Work out the finished part from the listing and answer in its coordinate system (mm). Face numbers are marked on the shaded views. A direction names the side the tool comes from. Round coordinates to 2 decimals unless told otherwise and drop trailing zeros. Order: outer loops, then holes, each group sorted by start corner. A loop starts at its lowest first (then second) coordinate and runs counter-clockwise, first axis right, second up. Notation, with made-up numbers: M 61.5,28.5 L 97.5,28.5 A22 ccw 97.5,58.5 Z; hole C 46,11 d11. An arc over 180 degrees is marked long. Return JSON: item names as keys, results as strings.
from build123d import *

# Parameters (mm, degrees)
SKETCH_1_R               = 14.75
EXTRUDE_1_DEPTH          = 20
SKETCH_2_R               = 14
EXTRUDE_2_DEPTH          = 5
SKETCH_3_R               = 14.75
EXTRUDE_3_DEPTH          = 5
SKETCH_4_R               = 14.25
SKETCH_4_R_2             = 13.5
EXTRUDE_4_DEPTH          = 6.7
SKETCH_5_R               = 13.5
EXTRUDE_5_DEPTH          = 6
SKETCH_6_W               = 1
SKETCH_6_H               = 10.048644724
CUT_EXTRUDE_1_DEPTH      = 15
PATTERN_CIRCULAR_1_COUNT = 24
SKETCH_7_R               = 1.5
EXTRUDE_6_DEPTH          = 17.7
SKETCH_8_R               = 10
EXTRUDE_7_DEPTH          = 1
SKETCH_9_R               = 13
EXTRUDE_8_DEPTH          = 3
SKETCH_10_R              = 8.9
EXTRUDE_9_DEPTH          = 3.3


with BuildPart() as part:
    # 草图1 → 凸台-拉伸1 (new body)
    with BuildSketch(Plane(origin=(0, 0, 0), x_dir=(0, 0, -1), z_dir=(1, 0, 0))):
        Circle(SKETCH_1_R)
    extrude(amount=EXTRUDE_1_DEPTH)

    # 草图2 → 凸台-拉伸2 (add)
    with BuildSketch(Plane(origin=(20, 0, 0), x_dir=(0, 0, -1), z_dir=(1, 0, 0))):
        Circle(SKETCH_2_R)
    extrude(amount=EXTRUDE_2_DEPTH)

    # 草图3 → 凸台-拉伸3 (add)
    with BuildSketch(Plane(origin=(25, 0, 0), x_dir=(0, 0, -1), z_dir=(1, 0, 0))):
        Circle(SKETCH_3_R)
    extrude(amount=EXTRUDE_3_DEPTH)

    # 草图4 → 凸台-拉伸4 (add)
    with BuildSketch(Plane(origin=(30, 0, 0), x_dir=(0, 0, -1), z_dir=(1, 0, 0))):
        Circle(SKETCH_4_R)
        Circle(SKETCH_4_R_2, mode=Mode.SUBTRACT)
    extrude(amount=EXTRUDE_4_DEPTH)

    # 草图5 → 凸台-拉伸5 (add)
    with BuildSketch(Plane(origin=(30, 0, 0), x_dir=(0, 0, -1), z_dir=(1, 0, 0))):
        Circle(SKETCH_5_R)
    extrude(amount=EXTRUDE_5_DEPTH)

    # 草图6 → 切除-拉伸1 (cut)
    with BuildSketch(Plane(origin=(36, 0, 0), x_dir=(0, 0, -1), z_dir=(1, 0, 0))):
        with Locations((0, 19.524322362)):
            Rectangle(SKETCH_6_W, SKETCH_6_H)
    cut_extrude_1 = extrude(amount=-CUT_EXTRUDE_1_DEPTH, mode=Mode.SUBTRACT)

    # 阵列(圆周)1: 切除-拉伸1 ×24 about axis
    pattern_circular_1_axis = Axis((0, 0, 0), (1, 0, 0))
    for i in range(1, PATTERN_CIRCULAR_1_COUNT):
        add(cut_extrude_1.rotate(pattern_circular_1_axis, i * 360 / PATTERN_CIRCULAR_1_COUNT), mode=Mode.SUBTRACT)

    # 草图7 → 凸台-拉伸6 (add)
    with BuildSketch(Plane(origin=(0, 0, 0), x_dir=(1, 0, 0), z_dir=(0, 1, 0))):
        with Locations(Location((3.8, 0, 0), (0, 0, 90))):
            Circle(SKETCH_7_R)
        with Locations(Location((16, 0, 0), (0, 0, 90))):
            Circle(SKETCH_7_R)
    extrude(amount=EXTRUDE_6_DEPTH)

    # 草图8 → 凸台-拉伸7 (add)
    with BuildSketch(Plane.ZY):
        Circle(SKETCH_8_R)
    extrude(amount=EXTRUDE_7_DEPTH)

    # 草图9 → 凸台-拉伸8 (add)
    with BuildSketch(Plane.ZY.offset(1)):
        Circle(SKETCH_9_R)
    extrude(amount=EXTRUDE_8_DEPTH)

    # 草图10 → 凸台-拉伸9 (add)
    with BuildSketch(Plane.ZY.offset(4)):
        Circle(SKETCH_10_R)
    extrude(amount=EXTRUDE_9_DEPTH)


solid = part.part
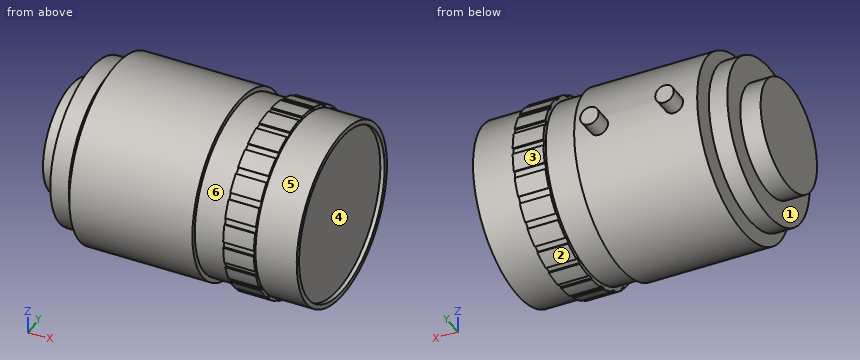
Item 1: Consider line 1 along Y through (x, z) = (36.35, 0); line 2 along X through (y, z) = (-10.5, 3.75); line 3 along X through (y, z) = (3, 6). Determine where each line is inside the solid, lowest interval first. Write a range as [from, to].
Output:
{"line 1": "y = [-14.25, -13.5], [13.5, 14.25]", "line 2": "x = [-4, -1], [0, 36]", "line 3": "x = [-7.3, 36]"}
Item 2: Find section C-C (x = -5). Determine the outline of the cut face in (y, z).
Output:
{"outline": "C 0,0 d17.8"}
Item 3: The mould has two halves that part along X. Classify the marked faces 4, 5 and 6: pulls with the +X half, pulls with the -X half, needs draft (parallel to the pull), parting line crosses it, or undercut.
Output:
{"face 4": "pulls with the +X half", "face 5": "needs draft", "face 6": "undercut"}
Item 4: Each of these flat-tipped pins is pushed along its axis until it touches: pin 1 (10 mm diameter, centred on x = 24.5, y = -9.5, fed in from -Z); pin 2 (8 mm diameter, centred on x = 11, z = 10, fed in from +Y); pin 3 (6 mm diameter, centred on x = 32, z = -8.5, fed in from +Y). Where does it stop, or does it pass through?
Output:
{"pin 1": "stops at z = -14.04", "pin 2": "stops at y = 13.47", "pin 3": "stops at y = 13.35"}
Item 5: Find section A-A (y = -11.5). Determine the outline of the cut face in (x, z), plus the area to 3 significant figures.
Output:
{"outline": "M -4,-6.06 L -1,-6.06 L -1,6.06 L -4,6.06 Z; M 0,-9.24 L 20,-9.24 L 20,-7.98 L 25,-7.98 L 25,-9.24 L 30,-9.24 L 30,-8.42 L 36.7,-8.42 L 36.7,-7.07 L 36,-7.07 L 36,7.07 L 36.7,7.07 L 36.7,8.42 L 30,8.42 L 30,9.24 L 25,9.24 L 25,7.98 L 20,7.98 L 20,9.24 L 0,9.24 Z", "area": "681 mm^2"}
Item 6: Which of the six approach directions +Z, -Z, +X, -X, +Y, -Y give full straight-line access (tool end or side, diameter ignored) to the marked faces 1, 2 and 3?
Output:
{"face 1": "-X", "face 2": "-Z, +X, -X, +Y", "face 3": "-Z, +X, +Y"}
